Input: part model. Units: mm. Frame: model coordinates. A direction names the side the tool comes from. Coordinates: 2 decimals unless noted, no trailing zeros. Write each loop counter-clockwise with the first axis right and the second up, starting at its lowest first coordinate (ties: lowest second). Pieces come first, ordered by that corner, then holes. Notation, with made-up numbers: M -32,7.5 L 8,7.5 A37 ccw 8,44.5 Z; hole C 33,19 d4. An arc over 180 degrees is marked long. Use CSV: the item, a comma, the result in double quotes.
```python
from build123d import *
from OCP.BRepFilletAPI import BRepFilletAPI_MakeChamfer

# Parameters (mm, degrees)
SKETCH2_W           = 144.5
SKETCH2_H           = 25
BOSS_EXTRUDE1_DEPTH = 8
SKETCH3_R           = 2.65
CUT_EXTRUDE1_DEPTH  = 74.758474089
SKETCH5_W           = 16
SKETCH5_H           = 25.5
SKETCH5_R           = 2.65
BOSS_EXTRUDE2_DEPTH = 8
FILLET1_R           = 5
FILLET2_R           = 2
CHAMFER1_SIZE       = 1
CHAMFER1_SIZE2      = 1.732050808
CHAMFER2_SIZE       = 1
CHAMFER2_SIZE2      = 0.577350269


with BuildPart() as part:
    # Sketch2 → Boss-Extrude1 (new body)
    with BuildSketch(Plane.XY):
        Rectangle(SKETCH2_W, SKETCH2_H)
    extrude(amount=BOSS_EXTRUDE1_DEPTH)

    # Sketch3 → Cut-Extrude1 (cut, through all)
    with BuildSketch(Plane.XY.offset(8)):
        with Locations((-60.25, 0)):
            Circle(SKETCH3_R)
        with Locations((60.25, 0)):
            Circle(SKETCH3_R)
    extrude(amount=-CUT_EXTRUDE1_DEPTH, mode=Mode.SUBTRACT)

    # Sketch5 → Boss-Extrude2 (add)
    # profile 1 of 2: a face of its own
    with BuildSketch(Plane.XY.offset(8)):
        with Locations((-30, -25.25)):
            Rectangle(SKETCH5_W, SKETCH5_H)
        with Locations((-30, -30)):
            Circle(SKETCH5_R, mode=Mode.SUBTRACT)
    # profile 2 of 2: a face of its own
    with BuildSketch(Plane.XY.offset(8)):
        with Locations((30, -25.25)):
            Rectangle(SKETCH5_W, SKETCH5_H)
        with Locations(Location((30, -30, 0), (0, 0, 180))):
            Circle(SKETCH5_R, mode=Mode.SUBTRACT)
    extrude(amount=-BOSS_EXTRUDE2_DEPTH)

    # Fillet1
    fillet1_edges = [part.edges().sort_by_distance(p)[0] for p in [
        (-38, -38, 4),
        (-38, -12.5, 4),
        (-22, -12.5, 4),
        (-22, -38, 4),
        (38, -12.5, 4),
        (38, -38, 4),
        (22, -38, 4),
        (22, -12.5, 4),
        (72.25, -12.5, 4),
        (-72.25, -12.5, 4),
        (-72.25, 12.5, 4),
        (72.25, 12.5, 4),
    ]]
    fillet(fillet1_edges, radius=FILLET1_R)

    # Fillet2
    fillet2_edges = [part.edges().sort_by_distance(p)[0] for p in [
        (38, -25.25, 8),
        (55.125, -12.5, 8),
        (30, -38, 8),
        (72.25, 0, 8),
        (0, 12.5, 8),
        (-72.25, 0, 8),
        (-55.125, -12.5, 8),
        (-38, -25.25, 8),
        (-30, -38, 8),
        (-22, -25.25, 8),
        (0, -12.5, 8),
        (22, -25.25, 8),
        (70.785533906, 11.035533906, 8),
        (70.785533906, -11.035533906, 8),
        (-70.785533906, 11.035533906, 8),
        (-70.785533906, -11.035533906, 8),
        (-23.464466094, -36.535533906, 8),
        (-36.535533906, -36.535533906, 8),
        (23.464466094, -36.535533906, 8),
        (36.535533906, -36.535533906, 8),
        (39.464466094, -13.964466094, 8),
        (20.535533906, -13.964466094, 8),
        (-39.464466094, -13.964466094, 8),
        (-20.535533906, -13.964466094, 8),
    ]]
    fillet(fillet2_edges, radius=FILLET2_R)

    # Chamfer1
    chamfer1_edges = [part.edges().sort_by_distance(p)[0] for p in [
        (38, -25.25, 0),
        (55.125, -12.5, 0),
        (30, -38, 0),
        (72.25, 0, 0),
        (22, -25.25, 0),
        (0, -12.5, 0),
        (-22, -25.25, 0),
        (-30, -38, 0),
        (-38, -25.25, 0),
        (-55.125, -12.5, 0),
        (-72.25, 0, 0),
        (0, 12.5, 0),
        (70.785533906, 11.035533906, 0),
        (70.785533906, -11.035533906, 0),
        (-70.785533906, 11.035533906, 0),
        (-70.785533906, -11.035533906, 0),
        (-23.464466094, -36.535533906, 0),
        (-36.535533906, -36.535533906, 0),
        (23.464466094, -36.535533906, 0),
        (36.535533906, -36.535533906, 0),
        (39.464466094, -13.964466094, 0),
        (20.535533906, -13.964466094, 0),
        (-39.464466094, -13.964466094, 0),
        (-20.535533906, -13.964466094, 0),
    ]]
    chamfer1_side = [part.faces().sort_by_distance(p)[0] for p in [
        (0, -4.348667021, 0),
    ]]
    chamfer(chamfer1_edges, length=CHAMFER1_SIZE, length2=CHAMFER1_SIZE2, reference=chamfer1_side[0])

    # Chamfer2: one chamfer whose edges measure the first distance from different faces: ONE call of the kernel's chamfer builder (chamfer() names one face for all edges)
    chamfer2_edges_1 = [part.edges().sort_by_distance(p)[0] for p in [
        (-62.9, 0, 0),
    ]]
    chamfer2_side_1 = [part.faces().sort_by_distance(p)[0] for p in [
        (-62.9, 0, 4),
    ]]
    chamfer2_edges_2 = [part.edges().sort_by_distance(p)[0] for p in [
        (57.6, 0, 0),
    ]]
    chamfer2_side_2 = [part.faces().sort_by_distance(p)[0] for p in [
        (57.6, 0, 4),
    ]]
    chamfer2_edges_3 = [part.edges().sort_by_distance(p)[0] for p in [
        (-32.65, -30, 0),
    ]]
    chamfer2_side_3 = [part.faces().sort_by_distance(p)[0] for p in [
        (-32.65, -30, 4),
    ]]
    chamfer2_edges_4 = [part.edges().sort_by_distance(p)[0] for p in [
        (32.65, -30, 0),
    ]]
    chamfer2_side_4 = [part.faces().sort_by_distance(p)[0] for p in [
        (32.65, -30, 4),
    ]]
    chamfer2 = BRepFilletAPI_MakeChamfer(part.part.solid().wrapped)
    for e in chamfer2_edges_1:
        chamfer2.Add(CHAMFER2_SIZE, CHAMFER2_SIZE2, e.wrapped, chamfer2_side_1[0].wrapped)  # the first distance lies on this face
    for e in chamfer2_edges_2:
        chamfer2.Add(CHAMFER2_SIZE, CHAMFER2_SIZE2, e.wrapped, chamfer2_side_2[0].wrapped)  # the first distance lies on this face
    for e in chamfer2_edges_3:
        chamfer2.Add(CHAMFER2_SIZE, CHAMFER2_SIZE2, e.wrapped, chamfer2_side_3[0].wrapped)  # the first distance lies on this face
    for e in chamfer2_edges_4:
        chamfer2.Add(CHAMFER2_SIZE, CHAMFER2_SIZE2, e.wrapped, chamfer2_side_4[0].wrapped)  # the first distance lies on this face
    add(Compound.cast(chamfer2.Shape()), mode=Mode.REPLACE)


solid = part.part
```
1. Section B-B (x = 60.25). Return loops of the section in (y, z).
Resolved:
outline,"M -12.5,1.73 L -11.5,0 L -3.23,0 L -2.65,1 L -2.65,8 L -10.5,8 A2 ccw -12.5,6 Z; M 2.65,1 L 3.23,0 L 11.5,0 L 12.5,1.73 L 12.5,6 A2 ccw 10.5,8 L 2.65,8 Z"
2. Material intervals for line 1 (X direction, y = -26, z = 2.25); line 2 (Y direction, x = 30, z = 3.25); line 3 (Y direction, x = -60.25, z = 6.25), sorted ascending. Write a range as [from, to].
Resolved:
line 1,"x = [-38, -22], [22, 38]"
line 2,"y = [-38, -32.65], [-27.35, 12.5]"
line 3,"y = [-12.48, -2.65], [2.65, 12.48]"
3. Section D-D (y = -30). Return loops of the section in (x, z).
Resolved:
outline,"M -38,1.73 L -37,0 L -33.23,0 L -32.65,1 L -32.65,8 L -36,8 A2 ccw -38,6 Z; M -27.35,1 L -26.77,0 L -23,0 L -22,1.73 L -22,6 A2 ccw -24,8 L -27.35,8 Z; M 22,1.73 L 23,0 L 26.77,0 L 27.35,1 L 27.35,8 L 24,8 A2 ccw 22,6 Z; M 32.65,1 L 33.23,0 L 37,0 L 38,1.73 L 38,6 A2 ccw 36,8 L 32.65,8 Z"
4. Section C-C (z = 4). Return loops of the section in (x, y), then the cut area to 3 significant figures.
Resolved:
outline,"M -72.25,-7.5 A5 ccw -67.25,-12.5 L -43,-12.5 A5 cw -38,-17.5 L -38,-33 A5 ccw -33,-38 L -27,-38 A5 ccw -22,-33 L -22,-17.5 A5 cw -17,-12.5 L 17,-12.5 A5 cw 22,-17.5 L 22,-33 A5 ccw 27,-38 L 33,-38 A5 ccw 38,-33 L 38,-17.5 A5 cw 43,-12.5 L 67.25,-12.5 A5 ccw 72.25,-7.5 L 72.25,7.5 A5 ccw 67.25,12.5 L -67.25,12.5 A5 ccw -72.25,7.5 Z; hole C -60.25,0 d5.3; hole C -30,-30 d5.3; hole C 30,-30 d5.3; hole C 60.25,0 d5.3"
area,"4,320 mm^2"
5. Contact query for flat-ended pins moving along their axis: pin 1 Ø3 at (x, y) = (-30, -30) entering from -Z; pin 2 Ø6 at (x, y) = (-30, -31) entering from +Z; pin 3 Ø1.3 at (x, z) = (-1, 3) entering from -Y; pin 4 Ø1 at (x, z) = (24.5, 4) entering from -Y. Output: stop coordinate, or through.
Resolved:
pin 1,"passes through"
pin 2,"stops at z = 8"
pin 3,"stops at y = -12.5"
pin 4,"stops at y = -37.58"
6. Mould query, pull axis X, two halves, no side actions, for faces 4 (the flat face through (-38, -25, 4)), 5 (the cylindrical face through (36, -37, 4)), 6 (the flat face through (55, -12.5, 4)), 7 (the conical face through (-23.926, -36.142, 0.686)). Classes: pulls with the +X half, pulls with the -X half, needs draft (parallel to the pull), parting line crosses it, or undercut.
Resolved:
face 4,"pulls with the -X half"
face 5,"pulls with the +X half"
face 6,"needs draft"
face 7,"undercut"
7. Section A-A (y = 0). Return loops of the section in (x, z), then the cut area to 3 significant figures.
Resolved:
outline,"M -72.25,1.73 L -71.25,0 L -63.48,0 L -62.9,1 L -62.9,8 L -70.25,8 A2 ccw -72.25,6 Z; M -57.6,1 L -57.02,0 L 57.02,0 L 57.6,1 L 57.6,8 L -57.6,8 Z; M 62.9,1 L 63.48,0 L 71.25,0 L 72.25,1.73 L 72.25,6 A2 ccw 70.25,8 L 62.9,8 Z"
area,"1,070 mm^2"
8. Access query for faces 1 (the cylindrical face through (-20.5, -13.93, 3.84)), 2 (the flat face through (38, -25, 4)), 3 (the flat face through (-30, -38, 4)). Directions: +Z, -Z, +X, -X, +Y, -Y. A direction counts if a zero-diameter tool reaches every point of the face in a straight line with its end or side. Return the directions, or none.
Resolved:
face 1,"+Z, -Z, -Y"
face 2,"+Z, -Z, +X, -Y"
face 3,"+Z, -Z, +X, -X, -Y"
